Model file for the job. Use its own axes, mm. Face numbers are marked on the shaded views. A direction names the side the tool comes from. Coordinates: 2 decimals unless noted, no trailing zeros. Order: outer loops, then holes, each group sorted by start corner. A loop starts at its lowest first (then second) coordinate and runs counter-clockwise, first axis right, second up. Notation, with made-up numbers: (77, 70) -> (82, 70) arc R21 ccw to (82, 104) -> close; hole circle Ø10 at (-34, 9.5). An arc over 180 degrees is marked (long way). Use CSV: the item, a comma, the result in double quotes. Start each with the question number.
(1) Cut at A-A on x = 0. Write the cut outline in (y, z).
(2) Tool access for the marked faces 1, 2, 3 and 4: list every direction of +Z, -Z, +X, -X, +Y, -Y with a clear straight run to the whole face (end or side of a thin tool).
(3) Cut at C-C on z = 47. Write the cut outline in (x, y), plus the area to 3 significant figures.
(4) Pin check, flat tips, straight feed: pin 1 Ø22 at (x, z) = (-18.5, 43.5) entering from +Y; pin 2 Ø3 at (y, z) = (0, -54) entering from -X; pin 3 Ø3 at (y, z) = (3, 53.5) entering from +X. Stop position of each tip, or through.
(5) Pull direction X, two halves, no side cores. Call the marked faces 5, 6 and 7: pulls with the +X half, pulls with the -X half, needs draft (parallel to the pull), parting line crosses it, or undercut.
(6) Probe L1, parallel to Z at x = -6, y = 5.5; L2, parallel to X at y = -4.5, z = 6.5; L3, parallel to Z at x = -16, y = 2. List the from-to ranges inside material, lowest first.
(7) Cut at B-B on x = -15. Write the cut outline in (y, z), plus the area to 3 significant figures.
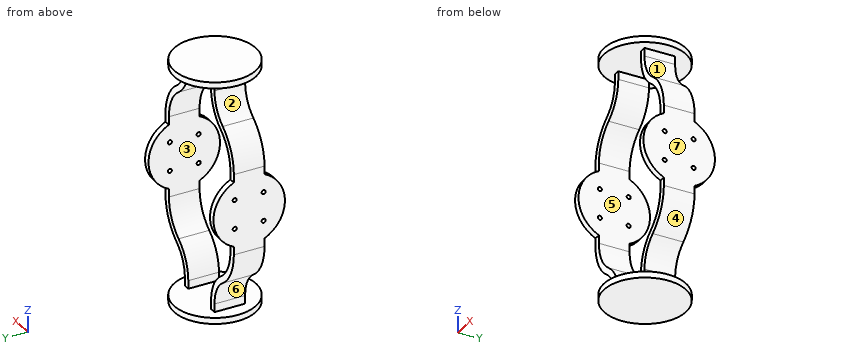
```python
from build123d import *

# Parameters (mm, degrees)
BOSS_EXTRUDE1_DEPTH = 25
SKETCH2_R           = 1
BOSS_EXTRUDE2_DEPTH = 25
SKETCH3_R           = 20
BOSS_EXTRUDE3_DEPTH = 3


with BuildPart() as part:
    # Sketch1 → Boss-Extrude1 (new, symmetric)
    with BuildSketch(Plane(origin=(0, 0, 0), x_dir=(1, 0, 0), z_dir=(0, 1, 0))):
        with BuildLine():
            Line((-27, -19.773863656), (-27, 19.773863656))
            ThreePointArc((-27, 19.773863656), (-24.748239349, 28.993408113), (-18.5, 36.136931828))
            ThreePointArc((-18.5, 36.136931828), (-12.251760651, 43.280455543), (-10, 52.5))
            Line((-10, 52.5), (-10, 59.5))
            Line((-10, 59.5), (-13, 59.5))
            Line((-13, 59.5), (-13, 52.5))
            ThreePointArc((-13, 52.5), (-14.913996553, 44.663387211), (-20.225, 38.591392054))
            ThreePointArc((-20.225, 38.591392054), (-27.410475252, 30.376339782), (-30, 19.773863656))
            Line((-30, 19.773863656), (-30, -19.773863656))
            ThreePointArc((-30, -19.773863656), (-27.410475252, -30.376339782), (-20.225, -38.591392054))
            ThreePointArc((-20.225, -38.591392054), (-14.913996553, -44.663387211), (-13, -52.5))
            Line((-13, -52.5), (-13, -59.5))
            Line((-13, -59.5), (-10, -59.5))
            Line((-10, -59.5), (-10, -52.5))
            ThreePointArc((-10, -52.5), (-12.251760651, -43.280455543), (-18.5, -36.136931828))
            ThreePointArc((-18.5, -36.136931828), (-24.748239349, -28.993408113), (-27, -19.773863656))
        make_face()
    extrude(amount=BOSS_EXTRUDE1_DEPTH, both=True)


with BuildPart() as body_2:
    # Sketch2 → Boss-Extrude2 (new, symmetric)
    with BuildSketch(Plane(origin=(-27, 0, 0), x_dir=(0, 0, -1), z_dir=(1, 0, 0))):
        with BuildLine():
            Line((15.811388301, -7.5), (59.5, -7.5))
            Line((59.5, -7.5), (59.5, 7.5))
            Line((59.5, 7.5), (15.811388301, 7.5))
            ThreePointArc((15.811388301, 7.5), (0, 17.5), (-15.811388301, 7.5))
            Line((-15.811388301, 7.5), (-59.5, 7.5))
            Line((-59.5, 7.5), (-59.5, -7.5))
            Line((-59.5, -7.5), (-15.811388301, -7.5))
            ThreePointArc((-15.811388301, -7.5), (0, -17.5), (15.811388301, -7.5))
        make_face()
        with Locations((7.071067812, -7.071067812)):
            Circle(SKETCH2_R, mode=Mode.SUBTRACT)
        with Locations((-7.071067812, -7.071067812)):
            Circle(SKETCH2_R, mode=Mode.SUBTRACT)
        with Locations((-7.071067812, 7.071067812)):
            Circle(SKETCH2_R, mode=Mode.SUBTRACT)
        with Locations((7.071067812, 7.071067812)):
            Circle(SKETCH2_R, mode=Mode.SUBTRACT)
    extrude(amount=BOSS_EXTRUDE2_DEPTH, both=True)

    # Combine1: intersect part
    add(part.part, mode=Mode.INTERSECT)


with BuildPart() as body_2_2:
    # Mirror3: mirrored copy
    add(body_2.part.mirror(Plane(origin=(0, 0, 0), x_dir=(0, 0, 1), z_dir=(1, 0, 0))))


with BuildPart() as body_2_1:
    add(body_2.part)

    add(body_2_2.part)  # Boss-Extrude3 merges body 2 2
    # Sketch3 → Boss-Extrude3 (add)
    with BuildSketch(Plane(origin=(0, 0, -59.5), x_dir=(-1, 0, 0), z_dir=(0, 0, -1))):
        Circle(SKETCH3_R)
    boss_extrude3 = extrude(amount=-BOSS_EXTRUDE3_DEPTH)

    # Mirror4: Boss-Extrude3 across plane
    add(boss_extrude3.mirror(Plane.XY))


solid = body_2_1.part
```
Outcome:
1,outline,"(-20, -59.5) -> (20, -59.5) -> (20, -56.5) -> (-20, -56.5) -> close; (-20, 56.5) -> (20, 56.5) -> (20, 59.5) -> (-20, 59.5) -> close"
2,face 1,"+X, +Y, -Y"
2,face 2,"-X, +Y, -Y"
2,face 3,"+Y, -Y"
2,face 4,"-Z, +X, +Y, -Y"
3,outline,"(-13.91, -7.5) -> (-10.77, -7.5) -> (-10.77, 7.5) -> (-13.91, 7.5) -> close; (10.77, -7.5) -> (13.91, -7.5) -> (13.91, 7.5) -> (10.77, 7.5) -> close"
3,area,"94.3 mm2"
4,pin 1,"y = 7.5"
4,pin 2,"x = -13"
4,pin 3,"x = 13.01"
5,face 5,"undercut"
5,face 6,"pulls with the -X half"
5,face 7,"pulls with the +X half"
6,L1,"-59.5 to -56.5, 56.5 to 59.5"
6,L2,"-30 to -27, 27 to 30"
6,L3,"-59.5 to -56.5, -42.86 to -38.22, 38.22 to 42.86, 56.5 to 59.5"
7,outline,"(-13.23, -59.5) -> (13.23, -59.5) -> (13.23, -56.5) -> (-13.23, -56.5) -> close; (-13.23, 56.5) -> (13.23, 56.5) -> (13.23, 59.5) -> (-13.23, 59.5) -> close; (-7.5, -44.5) -> (7.5, -44.5) -> (7.5, -39.27) -> (-7.5, -39.27) -> close; (-7.5, 39.27) -> (7.5, 39.27) -> (7.5, 44.5) -> (-7.5, 44.5) -> close"
7,area,"316 mm2"
